```python
from build123d import *

# Parameters (mm, degrees)
ESQUISSE1_W                   = 101.6
ESQUISSE1_H                   = 38.1
T_LE_DE_BASE_PLI_E1_DEPTH     = 4.76
ESQUISSE13_R                  = 4.7625
ENL_V_MAT_EXTRU_3_DEPTH       = 55.46283228
DIAM_TRE_DU_PER_AGE_5_0_5_1_D = 5
R_P_TITION_LIN_AIRE1_COUNT    = 2
R_P_TITION_LIN_AIRE1_PITCH    = 25.4
CONG_2_R                      = 3.175


# Sheet-metal steps are written as plain solids
with BuildPart() as part:
    # Esquisse1 → Tôle de base pliée1 (new body)
    with BuildSketch(Plane(origin=(0, 0, 0), x_dir=(1, 0, 0), z_dir=(0, 1, 0))):
        Rectangle(ESQUISSE1_W, ESQUISSE1_H)
    extrude(amount=-T_LE_DE_BASE_PLI_E1_DEPTH)

    # Esquisse13 → Enlèv. mat.-Extru.3 (cut, through all)
    with BuildSketch(Plane(origin=(0, 0, 0), x_dir=(1, 0, 0), z_dir=(0, 1, 0))):
        with Locations(Location((-39.8145, 0, 0), (0, 0, 270))):
            Circle(ESQUISSE13_R)
        with Locations(Location((39.8145, 0, 0), (0, 0, 90))):
            Circle(ESQUISSE13_R)
    extrude(amount=-ENL_V_MAT_EXTRU_3_DEPTH, mode=Mode.SUBTRACT)

    # Diamètre du perçage Ø5.0 (5)1 (through all)
    with Locations(Plane(origin=(0, 0, 0), x_dir=(1, 0, 0), z_dir=(0, 1, 0))):
        with Locations((-12.7, 12.7), (0, 12.7), (12.7, 12.7)):
            diam_tre_du_per_age_5_0_5_1 = Hole(DIAM_TRE_DU_PER_AGE_5_0_5_1_D / 2)

    # Répétition linéaire1: Diamètre du perçage Ø5.0 (5)1 ×2
    with Locations(*[(0, 0, i * R_P_TITION_LIN_AIRE1_PITCH) for i in range(1, R_P_TITION_LIN_AIRE1_COUNT)]):
        add(diam_tre_du_per_age_5_0_5_1, mode=Mode.SUBTRACT)

    # Congé2
    cong_2_edges = [part.edges().sort_by_distance(p)[0] for p in [
        (-50.8, -2.38, -19.05),
        (50.8, -2.38, -19.05),
        (50.8, -2.38, 19.05),
        (-50.8, -2.38, 19.05),
    ]]
    fillet(cong_2_edges, radius=CONG_2_R)


solid = part.part
```
The listing builds one solid part. Answer for the finished solid, in the listing's coordinates (mm). Coordinates: 2 decimals unless noted, no trailing zeros. Write each loop counter-clockwise with the first axis right and the second up, starting at its lowest first coordinate (ties: lowest second). Pieces come first, ordered by that corner, then holes. Notation, with made-up numbers: (9, 7.5) - (37, 7.5) arc R20 cw to (37, 17.5) - close; hole circle Ø6 at (-39.5, 3). An arc over 180 degrees is marked (long way). Return JSON: item names as keys, results as strings. Group by question number.
Q1. The part is cut by section A-A on z = 0. Write down the section's boundary in (x, y).
Q2. Find the intervals of material crossed by line 1 along X through (y, z) = (-3.15, 12.7); line 2 along Z through (x, y) = (12.7, -2.7); line 3 along X through (y, z) = (-1.85, -11.5), in increasing order. Write a range as [from, to].
Q3. For a pull along X with two mould halves and no side action, classify faces 1 (the cylindrical face through (49.85, -2.41, -18.14)), 2 (the cylindrical face through (-12.37, -2.41, -15.18)), 3 (the flat face through (-50.8, -2, 0)) as +X half, -X half, draft (parallel to the pull), parting line (faces both ways), or undercut.
Q4. The part is cut by section B-B on x = -12.7. Write down the section's boundary in (y, z).
Q5. The part is cut by section C-C on z = -12.7. Write down the section's boundary in (x, y).
Q6. The part is cut by section D-D on y = -2.6. State how many separate pieces and enclosed holes the cut face has, and give its area (3 significant figures).
Evaluation:
{
 "1": {"outline": "(-50.8, -4.76) - (-44.58, -4.76) - (-44.58, 0) - (-50.8, 0) - close; (-35.05, -4.76) - (35.05, -4.76) - (35.05, 0) - (-35.05, 0) - close; (44.58, -4.76) - (50.8, -4.76) - (50.8, 0) - (44.58, 0) - close"},
 "2": {"line 1": "x = [-50.8, -15.2], [-10.2, -2.5], [2.5, 10.2], [15.2, 50.8]", "line 2": "z = [-19.05, -15.2], [-10.2, 10.2], [15.2, 19.05]", "line 3": "x = [-50.8, -14.89], [-10.51, -2.19], [2.19, 10.51], [14.89, 50.8]"},
 "3": {"face 1": "+X half", "face 2": "undercut", "face 3": "-X half"},
 "4": {"outline": "(-4.76, -19.05) - (0, -19.05) - (0, -15.2) - (-4.76, -15.2) - close; (-4.76, -10.2) - (0, -10.2) - (0, 10.2) - (-4.76, 10.2) - close; (-4.76, 15.2) - (0, 15.2) - (0, 19.05) - (-4.76, 19.05) - close"},
 "5": {"outline": "(-50.8, -4.76) - (-15.2, -4.76) - (-15.2, 0) - (-50.8, 0) - close; (-10.2, -4.76) - (-2.5, -4.76) - (-2.5, 0) - (-10.2, 0) - close; (2.5, -4.76) - (10.2, -4.76) - (10.2, 0) - (2.5, 0) - close; (15.2, -4.76) - (50.8, -4.76) - (50.8, 0) - (15.2, 0) - close"},
 "6": {"separate pieces": "1", "enclosed holes": "8", "area": "3,600 mm2"}
}
